```python
from build123d import *

# Parameters (mm, degrees)
F0_R     = 20
F1_DEPTH = 0.7
F2_R     = 0.5
F3_DEPTH = 0.7


with BuildPart() as f1:
    # F0 (on Top) → F1 (new body)
    with BuildSketch(Plane.XY):
        Circle(F0_R)
    extrude(amount=F1_DEPTH)

    # F2 (on face) → F3 (cut)
    with BuildSketch(Plane.XY.offset(0.7)):
        with BuildLine():
            ThreePointArc((-4.646434, 4.646434), (-4.538048, 4.808646), (-4.499987, 4.999987))
            ThreePointArc((-4.499987, 4.999987), (-5.461927, 5.191329), (-4.646434, 4.646434))
        make_face()
        with BuildLine():
            ThreePointArc((5.499987, -4.999987), (5.191329, -4.538048), (4.646434, -4.646434))
            ThreePointArc((4.646434, -4.646434), (4.808646, -5.461927), (5.499987, -4.999987))
        make_face()
        with Locations((5.000013, 5.000013)):
            Circle(F2_R)
        with Locations((-5.000013, -5.000013)):
            Circle(F2_R)
        with Locations((-10.303288, 10.303288)):
            Circle(F2_R)
        with Locations((-8.535547, -8.535547)):
            Circle(F2_R)
        with Locations((7.170718, -7.070718)):
            Circle(F2_R)
        with Locations((11.902449, 12.235783)):
            Circle(F2_R)
    extrude(amount=-F3_DEPTH, mode=Mode.SUBTRACT)


solid = f1.part
```
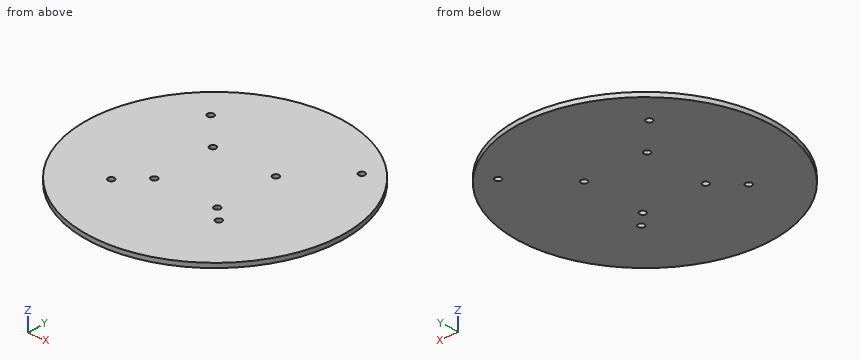
CAD build for the part. Positions are in the model's coordinates, mm. Give positions to 0.01 mm unless a question says otherwise; leave off trailing zeros. Write each loop counter-clockwise with the first axis right and the second up, starting at its lowest first coordinate (ties: lowest second). Pieces come first, ordered by that corner, then holes. Notation, with made-up numbers: M -15.75,76 L 43.25,76 A4 ccw 43.25,83 Z; hole C 40.5,13 d11. An arc over 180 degrees is marked long. Return JSON: item names as keys, results as strings. Group by question number.
(1) Band-saw the part on A-A (z = 0.35). State how many separate pieces and enclosed holes the cut face has, and give its area (3 significant figures).
(2) Drill centre lines: L1, parallel to Y at x = -10.5, z = 0.15; L2, parallel to Y at x = -8.5, z = 0.35; L3, parallel to X at y = 12, z = 0.2. Where is each one in solid material? Low to high. Write a range as [from, to].
(3) Band-saw the part on B-B (y = 4). Give the cut face in (x, z).
Entries:
{
 "1": {"separate pieces": "1", "enclosed holes": "8", "area": "1,250 mm^2"},
 "2": {"L1": "y = [-17.02, 9.84], [10.76, 17.02]", "L2": "y = [-18.1, -9.03], [-8.04, 18.1]", "L3": "x = [-16, 11.46], [12.34, 16]"},
 "3": {"outline": "M -19.6,0 L 19.6,0 L 19.6,0.7 L -19.6,0.7 Z"}
}
